from build123d import *

# Parameters (mm, degrees)
SCHIZZO1_W                   = 16
SCHIZZO1_H                   = 25
ESTRUSIONE_ESTRUSIONE1_DEPTH = 1.5
SCHIZZO2_R                   = 0.51
TAGLIO_ESTRUSIONE1_DEPTH     = 1.5
SCHIZZO3_W                   = 7
SCHIZZO3_H                   = 7
ESTRUSIONE_ESTRUSIONE2_DEPTH = 3


with BuildPart() as part:
    # Schizzo1 → Estrusione-Estrusione1 (new body)
    with BuildSketch(Plane(origin=(0, 0, 0), x_dir=(1, 0, 0), z_dir=(0, 1, 0))):
        with Locations((-8, 12.5)):
            Rectangle(SCHIZZO1_W, SCHIZZO1_H)
    extrude(amount=ESTRUSIONE_ESTRUSIONE1_DEPTH)

    # Schizzo2 → Taglio-Estrusione1 (cut)
    with BuildSketch(Plane(origin=(0, 1.5, 0), x_dir=(1, 0, 0), z_dir=(0, 1, 0))):
        with Locations(Location((-14.35, 23.73, 0), (0, 0, 270))):
            Circle(SCHIZZO2_R)
        with Locations(Location((-11.81, 23.73, 0), (0, 0, 270))):
            Circle(SCHIZZO2_R)
        with Locations(Location((-9.27, 23.73, 0), (0, 0, 270))):
            Circle(SCHIZZO2_R)
        with Locations(Location((-6.73, 23.73, 0), (0, 0, 270))):
            Circle(SCHIZZO2_R)
        with Locations(Location((-4.19, 23.73, 0), (0, 0, 270))):
            Circle(SCHIZZO2_R)
        with Locations(Location((-1.65, 23.73, 0), (0, 0, 270))):
            Circle(SCHIZZO2_R)
    extrude(amount=-TAGLIO_ESTRUSIONE1_DEPTH, mode=Mode.SUBTRACT)

    # Schizzo3 → Estrusione-Estrusione2 (add)
    with BuildSketch(Plane(origin=(0, 1.5, 0), x_dir=(1, 0, 0), z_dir=(0, 1, 0))):
        with Locations((-9.5, 16.5)):
            Rectangle(SCHIZZO3_W, SCHIZZO3_H)
    extrude(amount=ESTRUSIONE_ESTRUSIONE2_DEPTH)


solid = part.part
Geometry: final body of the model. Coordinates: model frame, mm. A direction names the side the tool comes from. Coordinates: 2 decimals unless noted, no trailing zeros. Order: outer loops, then holes, each group sorted by start corner. A loop starts at its lowest first (then second) coordinate and runs counter-clockwise, first axis right, second up.
1) Section B-B (z = -23.73). Return loops of the section in (x, y), then the cut area to 3 significant figures.
Result sheet:
outline: (-16, 0) - (-14.86, 0) - (-14.86, 1.5) - (-16, 1.5) - close; (-13.84, 0) - (-12.32, 0) - (-12.32, 1.5) - (-13.84, 1.5) - close; (-11.3, 0) - (-9.78, 0) - (-9.78, 1.5) - (-11.3, 1.5) - close; (-8.76, 0) - (-7.24, 0) - (-7.24, 1.5) - (-8.76, 1.5) - close; (-6.22, 0) - (-4.7, 0) - (-4.7, 1.5) - (-6.22, 1.5) - close; (-3.68, 0) - (-2.16, 0) - (-2.16, 1.5) - (-3.68, 1.5) - close; (-1.14, 0) - (0, 0) - (0, 1.5) - (-1.14, 1.5) - close
area: 14.8 mm2
2) Section D-D (y = 1.8). Return loops of the section in (x, z), then the cut area to 3 significant figures.
Result sheet:
outline: (-13, -20) - (-6, -20) - (-6, -13) - (-13, -13) - close
area: 49.0 mm2
3) Draft query along X for faces 6 (the cylindrical face through (-4.39, 0.76, -23.26)), 7 (the flat face through (-13, 3, -16)), 8 (the flat face through (-8, 1, 0)). Return one class per face: released by +X, released by -X, zero draft, split by the parting line, or undercut.
Result sheet:
face 6: undercut
face 7: released by -X
face 8: zero draft
4) First-contact query: P1, Ø1.5, axis at y = 3.5, z = -17, coming from the +X side; P2, Ø1.5, axis at x = -8, y = 2.5, coming from the +Z side; P3, Ø0.9, axis at x = -10, y = 3, coming from the -Z side. Flat tips, straight axial feed; report the tip coordinate or a pass-through.
Result sheet:
P1: stops at x = -6
P2: stops at z = -13
P3: stops at z = -20
5) Section C-C (x = -8.25). Return loops of the section in (y, z), then the cut area to 3 significant figures.
Result sheet:
outline: (0, -25) - (1.5, -25) - (1.5, -20) - (4.5, -20) - (4.5, -13) - (1.5, -13) - (1.5, 0) - (0, 0) - close
area: 58.5 mm2
6) Set-up query: faces 1 (the flat face through (-10, 3, -20)), 2 (the flat face through (-6, 3, -16)), 3 (the flat face through (-8, 0, -13)), 4 (the flat face through (-10, 3, -13)), 5 (the flat face through (-16, 1, -12)). Return all of +Z, -Z, +X, -X, +Y, -Y with unobstructed straight access to the full face (end or side cutting, diameter ignored); none if empty.
Result sheet:
face 1: -Z, +X, -X, +Y
face 2: +Z, -Z, +X, +Y
face 3: +Z, -Z, +X, -X, -Y
face 4: +Z, +X, -X, +Y
face 5: +Z, -Z, -X, +Y, -Y
7) Section A-A (x = -11.81). Return loops of the section in (y, z), then the cut area to 3 significant figures.
Result sheet:
outline: (0, -25) - (1.5, -25) - (1.5, -24.24) - (0, -24.24) - close; (0, -23.22) - (1.5, -23.22) - (1.5, -20) - (4.5, -20) - (4.5, -13) - (1.5, -13) - (1.5, 0) - (0, 0) - close
area: 57.0 mm2
8) Ray query, probe 1 along Y at (x, z) = (-3.5, -22.5); probe 2 along X at (y, z) = (2.65, -19); probe 3 along Z at (x, y) = (-12.5, 2.3). Return the intervals inside material, ascending.
Result sheet:
probe 1: y = 0 to 1.5
probe 2: x = -13 to -6
probe 3: z = -20 to -13
